```python
from build123d import *

# Parameters (mm, degrees)
EXTRUDE_1_DEPTH     = 42.3
SKETCH_2_R          = 11
SKETCH_2_R_2        = 1.5
SKETCH_2_R_3        = 2.5
CUT_EXTRUDE_1_DEPTH = 84.328146505
EXTRUDE_2_DEPTH     = 20
FILLET_1_R          = 2


with BuildPart() as part:
    # 스케치1 → 보스-돌출1 (new body)
    with BuildSketch(Plane(origin=(0, 0, 0), x_dir=(0, 0, -1), z_dir=(1, 0, 0))):
        Polygon((0, 5), (0, 0), (20, 0), (20, -20), (67.3, -20), (67.3, -15), (25, -15), (25, 5), align=None)
    extrude(amount=EXTRUDE_1_DEPTH)

    # 스케치2 → 컷-돌출1 (cut, through all)
    with BuildSketch(Plane(origin=(0, 5, 0), x_dir=(1, 0, 0), z_dir=(0, 1, 0))):
        Polygon((0, 61.65), (5.65, 67.3), (0, 67.3), align=None)
        Polygon((42.3, 67.3), (36.65, 67.3), (42.3, 61.65), align=None)
        with Locations(Location((21.15, 46.15, 0), (0, 0, 270))):
            Circle(SKETCH_2_R)
        with Locations(Location((5.65, 61.65, 0), (0, 0, 270))):
            Circle(SKETCH_2_R_2)
        with Locations(Location((36.65, 61.65, 0), (0, 0, 270))):
            Circle(SKETCH_2_R_2)
        with Locations(Location((5.65, 30.65, 0), (0, 0, 270))):
            Circle(SKETCH_2_R_2)
        with Locations(Location((36.65, 30.65, 0), (0, 0, 270))):
            Circle(SKETCH_2_R_2)
        with Locations(Location((10.575, 12.5, 0), (0, 0, 270))):
            Circle(SKETCH_2_R_3)
        with Locations(Location((31.725, 12.5, 0), (0, 0, 270))):
            Circle(SKETCH_2_R_3)
    extrude(amount=-CUT_EXTRUDE_1_DEPTH, mode=Mode.SUBTRACT)

    # 스케치2<4> → 보스-돌출2 (add)
    with BuildSketch(Plane(origin=(0, 5, 0), x_dir=(1, 0, 0), z_dir=(0, 1, 0))):
        Polygon((5.65, 25), (0, 30.65), (0, 25), align=None)
        Polygon((42.3, 25), (42.3, 30.65), (36.65, 25), align=None)
    extrude(amount=-EXTRUDE_2_DEPTH)

    # 필렛1
    fillet_1_edges = [part.edges().sort_by_distance(p)[0] for p in [
        (21.15, -20, -67.3),
        (42.3, -20, -40.825),
        (0, -20, -40.825),
        (21.15, -20, -20),
        (2.825, 5, -27.825),
        (21.15, 5, -25),
        (39.475, 5, -27.825),
        (21.15, 5, 0),
        (0, 5, -15.325),
        (42.3, 5, -15.325),
    ]]
    fillet(fillet_1_edges, radius=FILLET_1_R)


solid = part.part
```
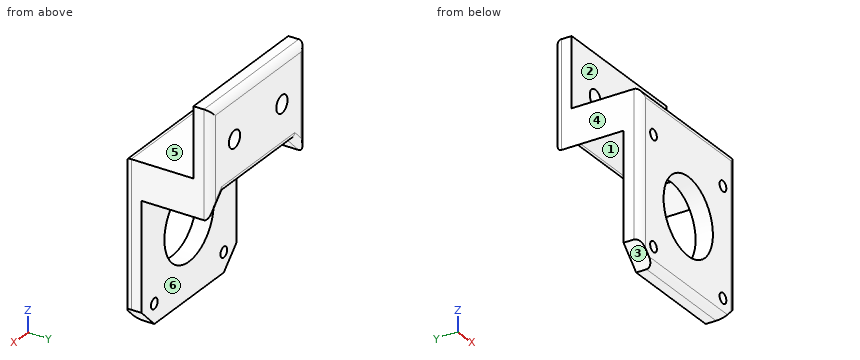
Part model, mm, in its own coordinate system. Face numbers are marked on the shaded views. A direction names the side the tool comes from. Round coordinates to 2 decimals unless told otherwise and drop trailing zeros. Write each loop counter-clockwise with the first axis right and the second up, starting at its lowest first coordinate (ties: lowest second). Pieces come first, ordered by that corner, then holes.
Item 1: Drop flat-ended pins along their axis: pin 1 Ø8 at (x, y) = (32, -11.5) entering from +Z; pin 2 Ø3.5 at (x, z) = (36.65, -61.65) entering from +Y; pin 3 Ø6 at (x, z) = (28, -5.5) entering from -Y. Give the stop position or say it passes through.
Results:
pin 1: stops at z = -20
pin 2: stops at y = -15
pin 3: stops at y = 0
Item 2: Cut at D-D, the plane z = -50. Give the cut face in (x, y), plus the area to 3 significant figures.
Results:
outline: (0, -18) arc R2 ccw to (2, -20) - (10.85, -20) - (10.85, -15) - (0, -15) - close; (31.45, -20) - (40.3, -20) arc R2 ccw to (42.3, -18) - (42.3, -15) - (31.45, -15) - close
area: 107 mm2
Item 3: Probe L1, parallel to X at y = -17.65, z = -30.65; L2, parallel to Y at x = 32, z = -3; L3, parallel to X at y = -18.7, z = -61.65. List the from-to ranges inside material, lowest first.
Results:
L1: x = 0 to 4.15, 7.15 to 35.15, 38.15 to 42.3
L2: y = 0 to 5
L3: x = 0.13 to 4.15, 7.15 to 35.15, 38.15 to 42.17
Item 4: Two-plate mould, pull along X, no slides. Class the marked faces 4, 5 and 6: +X half, -X half, draft (parallel to the pull), parting line (faces both ways), or undercut.
Results:
face 4: -X half
face 5: draft
face 6: undercut
Item 5: Cut at C-C, the plane y = -16. Give the cut face in (x, z), plus the area to 3 significant figures.
Results:
outline: (0, -61.65) - (5.65, -67.3) - (36.65, -67.3) - (42.3, -61.65) - (42.3, -20) - (0, -20) - close; hole circle Ø3 at (5.65, -61.65); hole circle Ø3 at (5.65, -30.65); hole circle Ø22 at (21.15, -46.15); hole circle Ø3 at (36.65, -61.65); hole circle Ø3 at (36.65, -30.65)
area: 1,560 mm2
Item 6: Cut at A-A, the plane x = 21.15. Give the cut face in (y, z).
Results:
outline: (-20, -65.3) arc R2 ccw to (-18, -67.3) - (-15, -67.3) - (-15, -57.15) - (-20, -57.15) - close; (-20, -35.15) - (-15, -35.15) - (-15, -25) - (3, -25) arc R2 ccw to (5, -23) - (5, -2) arc R2 ccw to (3, 0) - (0, 0) - (0, -20) - (-18, -20) arc R2 ccw to (-20, -22) - close
Item 7: Which spindle directions (+Z, -Z, +X, -X, +Y, -Y) get a long thin tool onto all of the face, cutting with end or side? Do the marked faces 1, 2 and 3. Say none if no direction does.
Results:
face 1: -Z, +Y
face 2: +Z, +X, -X, -Y
face 3: -Z, -X, +Y, -Y
Item 8: Cut at B-B, the plane z = -12.5. Give the cut face in (x, y) (3 decimals).
Results:
outline: (0, 0) - (8.075, 0) - (8.075, 5) - (2, 5) arc R2 ccw to (0, 3) - close; (13.075, 0) - (29.225, 0) - (29.225, 5) - (13.075, 5) - close; (34.225, 0) - (42.3, 0) - (42.3, 3) arc R2 ccw to (40.3, 5) - (34.225, 5) - close
